from build123d import *

# Parameters (mm, degrees)
SKETCH2_W           = 19.5
SKETCH2_H           = 20
BOSS_EXTRUDE1_DEPTH = 1.75
SKETCH3_W           = 19.5
SKETCH3_H           = 3.5
CUT_EXTRUDE1_DEPTH  = 2.75
SKETCH4_W           = 19.5
SKETCH4_H           = 1.75
BOSS_EXTRUDE2_DEPTH = 3.5
FILLET1_R           = 2
FILLET2_R           = 1


with BuildPart() as part:
    # Sketch1 → Revolve1 (revolve)
    with BuildSketch(Plane(origin=(0, 0, 0), x_dir=(0, 0, -1), z_dir=(1, 0, 0))):
        with BuildLine():
            Line((3, -6.873863542), (3, -16.25))
            Line((3, -16.25), (6, -16.25))
            Line((6, -16.25), (6, -18))
            Line((6, -18), (0, -18))
            Line((0, -18), (0, -7.5))
            Line((0, -7.5), (0, 7.5))
            ThreePointArc((0, 7.5), (7.341797347, 1.532322328), (3, -6.873863542))
        make_face()
    revolve(axis=Axis((0, 0, 0), (0, -1, 0)))

    # Sketch2 → Boss-Extrude1 (add)
    with BuildSketch(Plane.XZ.offset(18)):
        Rectangle(SKETCH2_W, SKETCH2_H)
    extrude(amount=-BOSS_EXTRUDE1_DEPTH)

    # Sketch3 → Cut-Extrude1 (cut, through all)
    with BuildSketch(Plane(origin=(0, -16.25, 0), x_dir=(1, 0, 0), z_dir=(0, 1, 0))):
        with Locations((0, -8.25)):
            Rectangle(SKETCH3_W, SKETCH3_H)
    extrude(amount=-CUT_EXTRUDE1_DEPTH, mode=Mode.SUBTRACT)

    # Sketch4 → Boss-Extrude2 (add)
    with BuildSketch(Plane(origin=(0, 0, -10), x_dir=(-1, 0, 0), z_dir=(0, 0, -1))):
        with Locations((0, -17.125)):
            Rectangle(SKETCH4_W, SKETCH4_H)
    extrude(amount=BOSS_EXTRUDE2_DEPTH)

    # Fillet1
    fillet1_edges = [part.edges().sort_by_distance(p)[0] for p in [
        (0, -6.873863542, 3),
    ]]
    fillet(fillet1_edges, radius=FILLET1_R)

    # Fillet2
    fillet2_edges = [part.edges().sort_by_distance(p)[0] for p in [
        (0, -16.25, 3),
    ]]
    fillet(fillet2_edges, radius=FILLET2_R)


solid = part.part
Part model, mm, in its own coordinate system. A direction names the side the tool comes from. Give positions to 0.01 mm unless a question says otherwise; leave off trailing zeros. Order: outer loops, then holes, each group sorted by start corner. A loop starts at its lowest first (then second) coordinate and runs counter-clockwise, first axis right, second up. Notation, with made-up numbers: (62.25, 67) -> (97.25, 67) arc R32 cw to (97.25, 103) -> close; hole circle Ø2 at (19, 72). An arc over 180 degrees is marked (long way). Use one line per item in the form item = value.
(1) Saw through at A-A (x = -7). Write the cut outline in (y, z).
Solution:
outline = (-18, -13.5) -> (-16.25, -13.5) -> (-16.25, 6.5) -> (-18, 6.5) -> close; circle Ø5.39 at (0, 0)
(2) Tool access for faces 1 (the face through (0, -17, 6.5)), 2 (the face through (9.75, -17, -3)): list every direction of +Z, -Z, +X, -X, +Y, -Y with a clear straight run to the whole face (end or side of a thin tool).
Solution:
face_1 = +Z, +X, -X, -Y
face_2 = +Z, -Z, +X, +Y, -Y
(3) Flat gauge pins, fed straight in: P1, Ø1.5, axis at y = -10, z = 4.5, coming from the +X side; P2, Ø8, axis at x = 3.5, y = 2, coming from the -Z side; P3, Ø0.9, axis at x = -1.5, y = -17.5, coming from the +Z side; P4, Ø1.5, axis at y = -5, z = 4.5, coming from the -X side. Where does each tip first touch, or does it go through?
Solution:
P1 = through
P2 = -7.5
P3 = 6.5
P4 = -4.53
(4) Drill centre lines: line 1 (Y direction, x = -0.5, z = -9); line 2 (Y direction, x = 1, z = 4); line 3 (Y direction, x = 1.25, z = 3.25). Where is each one in solid material? Low to high. Write a range as from..to.
Solution:
line_1 = -18..-16.25
line_2 = -18..-16.25, -6.26..6.26
line_3 = -18..-16.11, -6.78..6.64
(5) Saw through at C-C (y = 0). Write the cut outline in (x, z), then the cut area to 3 significant figures.
Solution:
outline = circle Ø15 at (0, 0)
area = 177 mm²
(6) Pull direction Y, two halves, no side cores. Call faces 3 (the face through (0.9, -11.71, -2.86)), 4 (the face through (0, -17, -13.5)), 5 (the face through (0, -18, -3)): +Y half, -Y half, draft (parallel to the pull), parting line (faces both ways), or undercut.
Solution:
face_3 = undercut
face_4 = draft
face_5 = -Y half
(7) Saw through at D-D (z = -10.25). Write the cut outline in (x, y).
Solution:
outline = (-9.75, -18) -> (9.75, -18) -> (9.75, -16.25) -> (-9.75, -16.25) -> close
(8) Saw through at B-B (z = 5.5). Write the cut outline in (x, y).
Solution:
outline = (-9.75, -18) -> (9.75, -18) -> (9.75, -16.25) -> (-9.75, -16.25) -> close; circle Ø10.2 at (0, 0)
